```python
from build123d import *

# Parameters (mm, degrees)
BASE_FLANGE1_DEPTH           = 2
EDGE_FLANGE1_STRIP_W         = 16
EDGE_FLANGE1_STRIP_H         = 2
EDGE_FLANGE1_STRIP_CUT_DEPTH = 900
EDGE_FLANGE1_DEPTH           = 900
EDGE_FLANGE2_STRIP_W         = 16
EDGE_FLANGE2_STRIP_H         = 2
EDGE_FLANGE2_STRIP_CUT_DEPTH = 894
EDGE_FLANGE2_DEPTH           = 894
EDGE_FLANGE3_START           = 4681.953522875
EDGE_FLANGE3_DEPTH           = 510.829009869
EDGE_FLANGE3_2_DEPTH         = 1
EDGE_FLANGE3_START_2         = 4682.953522875
EDGE_FLANGE3_3_DEPTH         = 509.829009869
EDGE_FLANGE4_START           = 228.014810269
EDGE_FLANGE4_DEPTH           = 482.051021673
EDGE_FLANGE4_2_DEPTH         = 1
EDGE_FLANGE4_START_2         = 229.014810269
EDGE_FLANGE4_3_DEPTH         = 481.051021673
SKETCH18_W                   = 34
SKETCH18_H                   = 43
CUT_EXTRUDE1_DEPTH           = 10
SKETCH19_W                   = 34
SKETCH19_H                   = 43
CUT_EXTRUDE2_DEPTH           = 10
SKETCH20_R                   = 4.25
CUT_EXTRUDE3_DEPTH           = 10
SKETCH21_R                   = 4.25
CUT_EXTRUDE4_DEPTH           = 10


# Read off the part's stored shape, not the designer's step: Edge-Flange3, Edge-Flange4
# Sheet-metal steps are written as plain solids
with BuildPart() as part:
    # Sketch1 → Base-Flange1 (new body)
    with BuildSketch(Plane(origin=(0, 0, 0), x_dir=(0, 0, -1), z_dir=(1, 0, 0))):
        with BuildLine():
            Line((-4682.953522875, -183.934168058), (-5198.782532744, -183.934168058))
            Line((-5198.782532744, -183.934168058), (-5198.782532744, 716.065831942))
            Line((-5198.782532744, 716.065831942), (-4298.782532744, 716.065831942))
            Line((-4298.782532744, 716.065831942), (-4298.782532744, 229.014810269))
            ThreePointArc((-4298.782532744, 229.014810269), (-4514.658558014, 44.672913809), (-4682.953522875, -183.934168058))
        make_face()
    extrude(amount=-BASE_FLANGE1_DEPTH)

    # Edge-Flange1 strip (across the edge) → Edge-Flange1 strip cut (cut)
    with BuildSketch(Plane(origin=(0, 716.065831942, 4298.782532744), x_dir=(0, -1, 0), z_dir=(0, 0, 1))):
        with Locations((-2, -1)):
            Rectangle(EDGE_FLANGE1_STRIP_W, EDGE_FLANGE1_STRIP_H)
    extrude(amount=EDGE_FLANGE1_STRIP_CUT_DEPTH, mode=Mode.SUBTRACT)

    # Edge-Flange1 section (across the edge) → Edge-Flange1 (add)
    with BuildSketch(Plane(origin=(0, 716.065831942, 4298.782532744), x_dir=(0, -1, 0), z_dir=(0, 0, 1))):
        with BuildLine():
            Line((0, 4), (0, 38))
            Line((0, 38), (2, 38))
            Line((2, 38), (2, 4))
            ThreePointArc((2, 4), (3.171572875, 1.171572875), (6, 0))
            Line((6, 0), (6, -2))
            ThreePointArc((6, -2), (1.757359313, -0.242640687), (0, 4))
        make_face()
    extrude(amount=EDGE_FLANGE1_DEPTH)

    # Edge-Flange2 strip (across the edge) → Edge-Flange2 strip cut (cut)
    with BuildSketch(Plane(origin=(0, 710.065831942, 5198.782532744), x_dir=(0, 0, -1), z_dir=(0, -1, 0))):
        with Locations((-2, -1)):
            Rectangle(EDGE_FLANGE2_STRIP_W, EDGE_FLANGE2_STRIP_H)
    extrude(amount=EDGE_FLANGE2_STRIP_CUT_DEPTH, mode=Mode.SUBTRACT)

    # Edge-Flange2 section (across the edge) → Edge-Flange2 (add)
    with BuildSketch(Plane(origin=(0, 710.065831942, 5198.782532744), x_dir=(0, 0, -1), z_dir=(0, -1, 0))):
        with BuildLine():
            Line((0, 4), (0, 38))
            Line((0, 38), (2, 38))
            Line((2, 38), (2, 4))
            ThreePointArc((2, 4), (3.171572875, 1.171572875), (6, 0))
            Line((6, 0), (6, -2))
            ThreePointArc((6, -2), (1.757359313, -0.242640687), (0, 4))
        make_face()
    extrude(amount=EDGE_FLANGE2_DEPTH)

    # Edge-Flange3 outline → Edge-Flange3 (cut)
    with BuildSketch(Plane.XY.offset(EDGE_FLANGE3_START)):
        with BuildLine():
            Line((0, -183.934168058), (0, -182.406304013))
            ThreePointArc((0, -182.406304013), (-1.477225575, -180.383657801), (-2, -177.934168058))
            Line((-2, -177.934168058), (-2, -183.934168058))
            Line((-2, -183.934168058), (0, -183.934168058))
        make_face()
    extrude(amount=EDGE_FLANGE3_DEPTH, mode=Mode.SUBTRACT)

    # Edge-Flange3 2 outline → Edge-Flange3 2 (cut)
    with BuildSketch(Plane.XY.offset(EDGE_FLANGE3_START)):
        with BuildLine():
            Line((0, -182.406304013), (0, -176.934168058))
            Line((0, -176.934168058), (-2, -176.934168058))
            Line((-2, -176.934168058), (-2, -177.934168058))
            ThreePointArc((-2, -177.934168058), (-1.477225575, -180.383657801), (0, -182.406304013))
        make_face()
    extrude(amount=EDGE_FLANGE3_2_DEPTH, mode=Mode.SUBTRACT)

    # Edge-Flange3 3 outline → Edge-Flange3 3 (add)
    with BuildSketch(Plane.XY.offset(EDGE_FLANGE3_START_2)):
        with BuildLine():
            Line((38, -183.934168058), (38, -181.934168058))
            Line((38, -181.934168058), (4, -181.934168058))
            ThreePointArc((4, -181.934168058), (1.171572875, -180.762595183), (0, -177.934168058))
            Line((0, -177.934168058), (0, -182.406304013))
            ThreePointArc((0, -182.406304013), (1.859067461, -183.539202212), (4, -183.934168058))
            Line((4, -183.934168058), (38, -183.934168058))
        make_face()
    extrude(amount=EDGE_FLANGE3_3_DEPTH)

    # Edge-Flange4 outline → Edge-Flange4 (cut)
    with BuildSketch(Plane(origin=(0, 0, 0), x_dir=(1, 0, 0), z_dir=(0, 1, 0)).offset(EDGE_FLANGE4_START)):
        with BuildLine():
            ThreePointArc((-2, -4304.782532744), (-1.477225575, -4302.333043001), (0, -4300.310396789))
            Line((0, -4300.310396789), (0, -4298.782532744))
            Line((0, -4298.782532744), (-2, -4298.782532744))
            Line((-2, -4298.782532744), (-2, -4304.782532744))
        make_face()
    extrude(amount=EDGE_FLANGE4_DEPTH, mode=Mode.SUBTRACT)

    # Edge-Flange4 2 outline → Edge-Flange4 2 (cut)
    with BuildSketch(Plane(origin=(0, 0, 0), x_dir=(1, 0, 0), z_dir=(0, 1, 0)).offset(EDGE_FLANGE4_START)):
        with BuildLine():
            Line((0, -4305.782532744), (0, -4300.310396789))
            ThreePointArc((0, -4300.310396789), (-1.477225575, -4302.333043001), (-2, -4304.782532744))
            Line((-2, -4304.782532744), (-2, -4305.782532744))
            Line((-2, -4305.782532744), (0, -4305.782532744))
        make_face()
    extrude(amount=EDGE_FLANGE4_2_DEPTH, mode=Mode.SUBTRACT)

    # Edge-Flange4 3 outline → Edge-Flange4 3 (add)
    with BuildSketch(Plane(origin=(0, 0, 0), x_dir=(1, 0, 0), z_dir=(0, 1, 0)).offset(EDGE_FLANGE4_START_2)):
        with BuildLine():
            Line((38, -4298.782532744), (4, -4298.782532744))
            ThreePointArc((4, -4298.782532744), (1.859067461, -4299.17749859), (0, -4300.310396789))
            Line((0, -4300.310396789), (0, -4304.782532744))
            ThreePointArc((0, -4304.782532744), (1.171572875, -4301.954105619), (4, -4300.782532744))
            Line((4, -4300.782532744), (38, -4300.782532744))
            Line((38, -4300.782532744), (38, -4298.782532744))
        make_face()
    extrude(amount=EDGE_FLANGE4_3_DEPTH)

    # Sketch18 → Cut-Extrude1 (cut)
    with BuildSketch(Plane.XZ.offset(183.934168058)):
        with Locations((21, 4704.453522875)):
            Rectangle(SKETCH18_W, SKETCH18_H)
    extrude(amount=-CUT_EXTRUDE1_DEPTH, mode=Mode.SUBTRACT)

    # Sketch19 → Cut-Extrude2 (cut)
    with BuildSketch(Plane(origin=(0, 0, 4298.782532744), x_dir=(-1, 0, 0), z_dir=(0, 0, -1))):
        with Locations((-21, 250.514810269)):
            Rectangle(SKETCH19_W, SKETCH19_H)
    extrude(amount=-CUT_EXTRUDE2_DEPTH, mode=Mode.SUBTRACT)

    # Sketch20 → Cut-Extrude3 (cut)
    with BuildSketch(Plane.XZ.offset(183.934168058)):
        with Locations((21, 5166.632532744)):
            Circle(SKETCH20_R)
        with Locations((21, 5041.632532744)):
            Circle(SKETCH20_R)
        with Locations((21, 4916.632532744)):
            Circle(SKETCH20_R)
        with Locations((21, 4791.632532744)):
            Circle(SKETCH20_R)
    extrude(amount=-CUT_EXTRUDE3_DEPTH, mode=Mode.SUBTRACT)

    # Sketch21 → Cut-Extrude4 (cut)
    with BuildSketch(Plane(origin=(0, 0, 4298.782532744), x_dir=(-1, 0, 0), z_dir=(0, 0, -1))):
        with Locations(Location((-21, 681.915831942, 0), (0, 0, 90))):
            Circle(SKETCH21_R)
        with Locations(Location((-21, 556.915831942, 0), (0, 0, 90))):
            Circle(SKETCH21_R)
        with Locations(Location((-21, 431.915831942, 0), (0, 0, 90))):
            Circle(SKETCH21_R)
        with Locations(Location((-21, 306.915831942, 0), (0, 0, 90))):
            Circle(SKETCH21_R)
    extrude(amount=-CUT_EXTRUDE4_DEPTH, mode=Mode.SUBTRACT)


solid = part.part
```
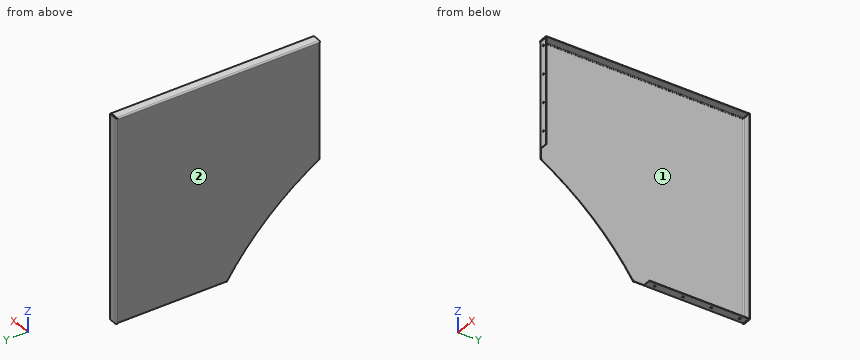
Build history of the part. All positions in model axes, mm. Face numbers are marked on the shaded views. Give positions to 0.01 mm unless a question says otherwise; leave off trailing zeros. Loops run counter-clockwise (first coordinate to the right, second up) from the corner with the lowest first, then second, coordinate; pieces in that order, holes last.
Item 1: Drill centre lines: line 1 (Z direction, x = 21, y = -183.25); line 2 (Y direction, x = 25, z = 4838); line 3 (Z direction, x = 18, y = 603.5). Where is each one in solid material? Low to high.
Answers follow:
line 1: z = 4725.95 to 4787.38, 4795.88 to 4912.38, 4920.88 to 5037.38, 5045.88 to 5162.38, 5170.88 to 5192.78, 5196.78 to 5198.78
line 2: y = -183.93 to -181.93, 714.07 to 716.07
line 3: z = 4298.78 to 4300.78, 5196.78 to 5198.78
Item 2: Slice it at D-D, the plane y = -88.5. List the corners of the cut face in (x, z), and give its area (3 significant figures).
Answers follow:
outline: (-2, 4622.39) - (0, 4622.39) - (0, 5192.78) arc R4 cw to (4, 5196.78) - (38, 5196.78) - (38, 5198.78) - (4, 5198.78) arc R6 ccw to (-2, 5192.78) - close
area: 1,220 mm2
Item 3: Slice it at C-C, the plane z = 5062. List the corners of the cut face in (x, y).
Answers follow:
outline: (-2, -177.93) arc R6 ccw to (4, -183.93) - (38, -183.93) - (38, -181.93) - (4, -181.93) arc R4 cw to (0, -177.93) - (0, 710.07) arc R4 cw to (4, 714.07) - (38, 714.07) - (38, 716.07) - (4, 716.07) arc R6 ccw to (-2, 710.07) - close
Item 4: Pull direction Z, two halves, no side cores. Call the marked faces 1 and 2: released by +Z, released by -Z, zero draft, split by the parting line, or undercut.
Answers follow:
face 1: undercut
face 2: zero draft
Item 5: Slice it at B-B, the plane y = 328.5. List the corners of the cut face in (x, z).
Answers follow:
outline: (-2, 4304.78) arc R6 ccw to (4, 4298.78) - (38, 4298.78) - (38, 4300.78) - (4, 4300.78) arc R4 cw to (0, 4304.78) - (0, 5192.78) arc R4 cw to (4, 5196.78) - (38, 5196.78) - (38, 5198.78) - (4, 5198.78) arc R6 ccw to (-2, 5192.78) - close
Item 6: Slice it at A-A, the plane x = 31.5. List the corners of the cut face in (y, z), and give its area (3 significant figures).
Answers follow:
outline: (-183.93, 4725.95) - (-181.93, 4725.95) - (-181.93, 5192.78) - (-183.93, 5192.78) - close; (-183.93, 5196.78) - (710.07, 5196.78) - (710.07, 5198.78) - (-183.93, 5198.78) - close; (272.01, 4298.78) - (710.07, 4298.78) - (710.07, 4300.78) - (272.01, 4300.78) - close; (714.07, 4298.78) - (716.07, 4298.78) - (716.07, 5198.78) - (714.07, 5198.78) - close
area: 5,400 mm2
Item 7: Flat gauge pins, fed straight in: pin 1 (8 mm diameter, centred on x = 16.5, z = 4456, fed in from -Y); pin 2 (1.6 mm diameter, centred on y = -183.5, z = 4714, fed in from +X); pin 3 (2 mm diameter, centred on x = 22, z = 4300, fed in from -Y). Where does each tip first touch, or does it go through?
Answers follow:
pin 1: stops at y = 714.07
pin 2: stops at x = 4
pin 3: stops at y = 272.01
